Part model, mm, in its own coordinate system. A direction names the side the tool comes from. Give positions to 0.01 mm unless a question says otherwise; leave off trailing zeros. Order: outer loops, then holes, each group sorted by start corner. A loop starts at its lowest first (then second) coordinate and runs counter-clockwise, first axis right, second up. Notation, with made-up numbers: (72.25, 32) -> (84.25, 32) arc R33 ccw to (84.25, 65) -> close; hole circle Ø10 at (76, 81.25). An arc over 180 degrees is marked (long way). Write item = value, one per line. Start each with the question number.
Item 1: Flat gauge pins, fed straight in: P1, Ø0.9, axis at x = 55, z = 13.5, coming from the -Y side; P2, Ø3.5, axis at x = 44.5, z = 9, coming from the +Y side; P3, Ø1.5, axis at x = 87.5, z = 42.5, coming from the +Y side; P4, Ø0.9, axis at x = 45, y = 9.5, coming from the -Z side. Where does each tip first touch, or does it go through?
Item 2: Tool access for faces 4 (the face through (55, 8.5, 10)), 5 (the face through (49, 0, 39)), 6 (the face through (11.5, 115, 32)): list every direction of +Z, -Z, +X, -X, +Y, -Y with a clear straight run to the whole face (end or side of a thin tool).
Item 3: Band-saw the part on A-A on z = 31. Write the cut outline in (x, y) (3 decimals).
Item 4: Band-saw the part on B-B on z = 12.5. Write the cut outline in (x, y).
Item 5: Pull direction X, two halves, no side cores. Call faces 1 (the face through (55, 10, 20)), 2 (the face through (0, 64, 41)), 3 (the face through (51, 49, 80)): +X half, -X half, draft (parallel to the pull), parting line (faces both ways), or undercut.
Item 6: Drill centre lines: line 1 along Y through (x, z) = (15, 66); line 2 along Y through (x, z) = (70, 5) (3 decimals). Where is each one in solid material? Low to high.
Autodesk Fusion 360 part; units mm, degrees
sketch "Sketch1" plane through (0, 0, 0) normal (0, 1, 0) x (1, 0, 0)
  line L0 (0, 0) -> (100, 0)
  line L1 (100, 0) -> (100, -80)
  line L2 (100, -80) -> (0, -80)
  line L3 (0, -80) -> (0, 0)
  dimension "d1" = 100
  dimension "d2" = 80
extrude "Extrude1" add sketch "Sketch1" along normal blind 130
sketch "Sketch2" plane through (100, 0, 0) normal (1, 0, 0) x (0, 0, -1)
  line L0 (-80, 0) -> (0, 0)
  line L1 (0, 0) -> (0, 130)
  line L2 (0, 130) -> (-80, 130)
  line L3 (-80, 130) -> (-80, 0)
  line L4 (-80, 130) -> (-80, 100)
  line L5 (-80, 100) -> (0, 130)
extrude "Extrude2" cut sketch "Sketch2" against normal blind 130 contours L2 L3 L4 L5
sketch "Sketch3" plane through (0, 113.9726, 42.7397) normal (0, 0.9363, 0.3511) x (1, 0, 0)
  line L0 (0, 45.646) -> (0, -39.794)
  line L1 (0, -39.794) -> (100, -39.794)
  line L2 (100, -39.794) -> (100, 45.646)
  line L3 (100, 45.646) -> (0, 45.646)
  line L4 (11.5, 35.646) -> (88.5, 35.646)
  line L5 (88.5, 35.646) -> (88.5, -14.354)
  line L6 (88.5, -14.354) -> (11.5, -14.354)
  line L7 (11.5, -14.354) -> (11.5, 35.646)
  circle A0 centre (50, -27.074) radius 6
  dimension "d7" = 50
  dimension "d8" = 77
  dimension "d9" = 11.5
  dimension "d10" = 19.8322
  dimension "d11" = 10
  dimension "d12" = 25.44
  dimension "d13" = 12.72
  dimension "d14" = 50
  dimension "d15" = 12
extrude "Extrude4" cut sketch "Sketch3" against normal blind 40 contours A0
extrude "Extrude3" cut sketch "Sketch3" against normal blind 6 contours L4 L5 L6 L7
sketch "Sketch4" plane through (0, 0, 0) normal (0, 0, -1) x (-1, 0, 0)
  line L0 (-100, 0) -> (0, 0)
  line L1 (0, 0) -> (0, 130)
  line L2 (0, 130) -> (-100, 130)
  line L3 (-100, 130) -> (-100, 0)
  line L4 (-56.5, 11.5) -> (-53.5, 11.5)
  line L5 (-53.5, 11.5) -> (-53.5, 8.5)
  line L6 (-53.5, 8.5) -> (-56.5, 8.5)
  line L7 (-56.5, 8.5) -> (-56.5, 11.5)
  line L8 (-56.5, 11.5) -> (-53.5, 8.5) construction
  line L9 (-53.5, 11.5) -> (-56.5, 8.5) construction
  line L10 (-46.5, 11.5) -> (-43.5, 11.5)
  line L11 (-43.5, 11.5) -> (-43.5, 8.5)
  line L12 (-43.5, 8.5) -> (-46.5, 8.5)
  line L13 (-46.5, 8.5) -> (-46.5, 11.5)
  line L14 (-46.5, 11.5) -> (-43.5, 8.5) construction
  line L15 (-43.5, 11.5) -> (-46.5, 8.5) construction
  dimension "d20" = 10
  dimension "d21" = 10
  dimension "d22" = 3
  dimension "d23" = 3
  dimension "d24" = 3
  dimension "d25" = 3
  dimension "d30" = 45
extrude "Extrude7" cut sketch "Sketch4" against normal blind 20 contours L4 L5 L6 L7
extrude "Extrude5" cut sketch "Sketch4" against normal blind 14 contours L4 L5 L6 L7
extrude "Extrude6" cut sketch "Sketch4" against normal blind 18 contours L10 L11 L12 L13
equation "d13 = ( 25.44 / 2 ) * 1 mm"
Values found:
q1.P1 = 0
q1.P2 = 127.28
q1.P3 = 114.34
q1.P4 = 18
q2.face_4 = -Z
q2.face_5 = +Z, -Z, +X, -X, -Y
q2.face_6 = none
q3.outline = (0, 0) -> (100, 0) -> (100, 118.375) -> (0, 118.375) -> close; hole (11.5, 111.967) -> (88.5, 111.967) -> (88.5, 118.375) -> (11.5, 118.375) -> close
q4.outline = (0, 0) -> (100, 0) -> (100, 125.31) -> (0, 125.31) -> close; hole (11.5, 118.9) -> (88.5, 118.9) -> (88.5, 125.31) -> (11.5, 125.31) -> close; hole (43.5, 8.5) -> (46.5, 8.5) -> (46.5, 11.5) -> (43.5, 11.5) -> close; hole (53.5, 8.5) -> (56.5, 8.5) -> (56.5, 11.5) -> (53.5, 11.5) -> close
q5.face_1 = undercut
q5.face_2 = -X half
q5.face_3 = draft
q6.line_1 = 0 to 105.25
q6.line_2 = 0 to 128.125
